from build123d import *

# Parameters (mm, degrees)
SKETCH_1_W          = 30
SKETCH_1_H          = 24
EXTRUDE_1_DEPTH     = 20
CUT_EXTRUDE_1_DEPTH = 15
CUT_EXTRUDE_2_DEPTH = 39


with BuildPart() as part:
    # 草圖1 → 填料-伸長1 (new body)
    with BuildSketch(Plane.XY):
        Rectangle(SKETCH_1_W, SKETCH_1_H)
    extrude(amount=-EXTRUDE_1_DEPTH)

    # 草圖2 → 除料-伸長1 (cut)
    with BuildSketch(Plane(origin=(0, 12, 0), x_dir=(1, 0, 0), z_dir=(0, 1, 0))):
        Polygon((0, 0), (0, 20), (-5, 20), (-10, 0), align=None)
        Polygon((10, 0), (5, 20), (0, 20), (0, 0), align=None)
    extrude(amount=-CUT_EXTRUDE_1_DEPTH, mode=Mode.SUBTRACT)

    # 草圖3 → 除料-伸長2 (cut, through all)
    with BuildSketch(Plane(origin=(15, 0, 0), x_dir=(0, 0, -1), z_dir=(1, 0, 0))):
        Polygon((0, -7), (20, 12), (0, 12), align=None)
    extrude(amount=-CUT_EXTRUDE_2_DEPTH, mode=Mode.SUBTRACT)


solid = part.part
CAD build for the part. Positions are in the model's coordinates, mm. A direction names the side the tool comes from. Give positions to 0.01 mm unless a question says otherwise; leave off trailing zeros. Order: outer loops, then holes, each group sorted by start corner. A loop starts at its lowest first (then second) coordinate and runs counter-clockwise, first axis right, second up. Notation, with made-up numbers: (49, 9.25) - (53, 9.25) arc R22 cw to (53, 43.25) - close; hole circle Ø5 at (45.5, 43.25). An arc over 180 degrees is marked (long way). Answer in a Markdown table with one row per item.
1. Saw through at C-C, the plane z = -16.75. Give the cut face in (x, y).
Data:
| item | result |
|---|---|
| outline | (-15, -12) - (15, -12) - (15, 8.91) - (5.81, 8.91) - (5.81, -3) - (-5.81, -3) - (-5.81, 8.91) - (-15, 8.91) - close |
2. Probe probe 1 along Y at (x, z) = (-0.5, -12.5); probe 2 along Y at (x, z) = (-14, -10); probe 3 along X at (y, z) = (-1.5, -14.75). List the from-to ranges inside material, lowest first. Write a range as [from, to].
Data:
| item | result |
|---|---|
| probe 1 | y = [-12, -3] |
| probe 2 | y = [-12, 2.5] |
| probe 3 | x = [-15, -6.31], [6.31, 15] |
3. Saw through at D-D, the plane y = 8.5. Give the cut face in (x, z).
Data:
| item | result |
|---|---|
| outline | (-15, -20) - (-5, -20) - (-5.92, -16.32) - (-15, -16.32) - close; (5, -20) - (15, -20) - (15, -16.32) - (5.92, -16.32) - close |
4. Saw through at A-A, the plane y = 2.5. Give the cut face in (x, z).
Data:
| item | result |
|---|---|
| outline | (-15, -20) - (-5, -20) - (-7.5, -10) - (-15, -10) - close; (5, -20) - (15, -20) - (15, -10) - (7.5, -10) - close |
5. Tool access for faces 4 (the flat face through (0, -9, 0)), 5 (the flat face through (0, -3, -12)): list every direction of +Z, -Z, +X, -X, +Y, -Y with a clear straight run to the whole face (end or side of a thin tool).
Data:
| item | result |
|---|---|
| face 4 | +Z, +X, -X, +Y, -Y |
| face 5 | +Z, +Y |
6. Pull direction X, two halves, no side cores. Call faces 1 (the flat face through (0, -5, -20)), 2 (the flat face through (15, -3, -12)), 3 (the flat face through (6, 1, -16)): pulls with the +X half, pulls with the -X half, needs draft (parallel to the pull), parting line crosses it, or undercut.
Data:
| item | result |
|---|---|
| face 1 | needs draft |
| face 2 | pulls with the +X half |
| face 3 | undercut |
7. Flat gauge pins, fed straight in: pin 1 (12 mm diameter, centred on x = -1, z = -10.5, fed in from +Y); pin 2 (1.5 mm diameter, centred on y = 7.5, z = -12.5, fed in from -X). Where does each tip first touch, or does it go through?
Data:
| item | result |
|---|---|
| pin 1 | stops at y = -3 |
| pin 2 | passes through |
8. Saw through at B-B, the plane x = -7. Give the cut face in (y, z).
Data:
| item | result |
|---|---|
| outline | (-12, -20) - (12, -20) - (4.4, -12) - (-3, -12) - (-3, -4.21) - (-7, 0) - (-12, 0) - close |
